The model under review builds one solid part; all positions refer to its coordinate system, in mm. Face numbers are marked on the shaded views. Round coordinates to 2 decimals unless told otherwise and drop trailing zeros. Write each loop counter-clockwise with the first axis right and the second up, starting at its lowest first coordinate (ties: lowest second). Pieces come first, ordered by that corner, then holes. Notation, with made-up numbers: (66, -6) -> (108, -6) arc R13 cw to (108, -1) -> close; hole circle Ø8 at (-22.75, 81). An arc over 180 degrees is marked (long way). Use CSV: the item, a comma, the result in double quotes. Start each with the question number.
1) For pin 1 Ø2 at (y, z) = (-2.5, -1.5) entering from +X, flat-tipped, find the tip position at first contact; note if it passes through.
2) Mouldability with a two-part tool opening along X and no side actions: class the marked faces 1, 2 and 3 as released by +X, released by -X, zero draft, split by the parting line, or undercut.
3) Wall thickness on probe 1 along X at (y, z) = (-4.95, 0); probe 2 along Y at (x, z) = (-3, 6); probe 3 along X at (y, z) = (-1.9, 7): over which ranges is each line inside the solid? List them lowest first. Write a range as [from, to].
4) Take a section at C-C, the plane y = -2.7. Give the boundary of the cut face in (x, z), then the cut area to 3 significant figures.
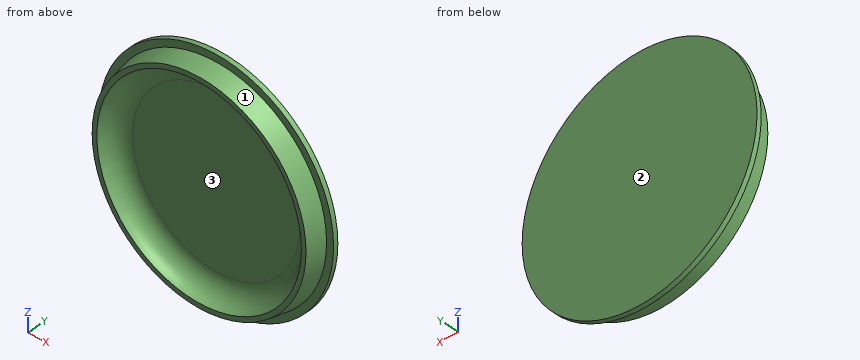
from build123d import *

# Parameters (mm, degrees)
FILLET1_R = 4


with BuildPart() as part:
    # Sketch2 → Revolve3 (revolve)
    with BuildSketch(Plane.XY):
        Polygon((22, -5), (22, -1), (0, -1), (0, 0), (25.25, 0), (25.25, -1), (23.75, -1), (23, -5), align=None)
    revolve(axis=Axis((0, -1, 0), (0, 1, 0)))

    # Fillet1
    fillet1_edges = [part.edges().sort_by_distance(p)[0] for p in [
        (-22, -1, 0),
    ]]
    fillet(fillet1_edges, radius=FILLET1_R - 0.0001)  # a hair under: the kernel refuses the full size


solid = part.part
Values found:
1,pin 1,"x = 23.62"
2,face 1,"split by the parting line"
2,face 2,"zero draft"
2,face 3,"undercut"
3,probe 1,"[-23.01, -22], [22, 23.01]"
3,probe 2,"[-1, 0]"
3,probe 3,"[-22.52, -19.3], [19.3, 22.52]"
4,outline,"circle Ø46.86 at (0, 0); hole circle Ø42.55 at (0, 0)"
4,area,"303 mm²"
